Geometry: final body of the model. Coordinates: model frame, mm. A direction names the side the tool comes from. Round coordinates to 2 decimals unless told otherwise and drop trailing zeros. Loops run counter-clockwise (first coordinate to the right, second up) from the corner with the lowest first, then second, coordinate; pieces in that order, holes last. Notation, with made-up numbers: M 75.25,-38.5 L 107.25,-38.5 A33 ccw 107.25,-4.5 Z; hole C 79,75.25 d6. An arc over 180 degrees is marked long. Answer as a JSON object with one key per item and string values.
```python
from build123d import *

# Parameters (mm, degrees)
F1_DEPTH = 100
F2_W     = 980
F2_H     = 769.125695
F3_DEPTH = 250
F4_W     = 244.644434
F4_H     = 193.814576
F4_W_2   = 221.683964
F4_H_2   = 205.729261
F5_DEPTH = 600


with BuildPart() as f1:
    # F0 (on Top) → F1 (new body)
    with BuildSketch(Plane.XY):
        Polygon((-780, 0), (0, 0), (-18.731487, 589.702579), (-748.441424, 569.125695), align=None)
    extrude(amount=F1_DEPTH)

    # F2 (on face) → F3 (join)
    with BuildSketch(Plane(origin=(0, 0, 0), x_dir=(1, 0, 0), z_dir=(0, 0, -1))):
        with Locations((-390, -284.562847)):
            Rectangle(F2_W, F2_H)
    extrude(amount=F3_DEPTH)

    # F4 (on face) → F5 (cut)
    with BuildSketch(Plane.XY.offset(100)):
        with Locations((-537.912771, 294.744283)):
            Rectangle(F4_W, F4_H)
        with Locations((-218.167432, 298.055314)):
            Rectangle(F4_W_2, F4_H_2)
    extrude(amount=-F5_DEPTH, mode=Mode.SUBTRACT)


solid = f1.part
```
1) First-contact query: pin 1 (6 mm diameter, centred on y = 254.5, z = 60.5, fed in from +X); pin 2 (10 mm diameter, centred on y = 201, z = 47.5, fed in from -X); pin 3 (4 mm diameter, centred on y = -1.5, z = 21, fed in from -X). Flat tips, straight axial feed; report the tip coordinate or a pass-through.
Geometry results:
{"pin 1": "x = -7.99", "pin 2": "x = -769.13", "pin 3": "x = -780"}
2) Cut plane C-C on y = 295. Return the cut outline in (x, z), and give its area (3 significant figures).
Geometry results:
{"outline": "M -880,-250 L -660.23,-250 L -660.23,100 L -763.64,100 L -763.64,0 L -880,0 Z; M -415.59,-250 L -329.01,-250 L -329.01,100 L -415.59,100 Z; M -107.33,-250 L 100,-250 L 100,0 L -9.37,0 L -9.37,100 L -107.33,100 Z", "area": "157,000 mm2"}
3) Set-up query: faces 5 (the face through (-395, 0, 49)), 6 (the face through (-764, 288.55, 49.3)), 7 (the face through (-660.235, 293, -73)), 8 (the face through (100, 290, -123)), 9 (the face through (-397, -100, -123)). Return all of +Z, -Z, +X, -X, +Y, -Y with unobstructed straight access to the full face (end or side cutting, diameter ignored); none if empty.
Geometry results:
{"face 5": "+Z, +X, -X, -Y", "face 6": "+Z, -X, +Y", "face 7": "+Z, -Z", "face 8": "+Z, -Z, +X, +Y, -Y", "face 9": "+Z, -Z, +X, -X, -Y"}
4) Cut plane D-D on x = -728. Return the cut outline in (y, z), and give its area (3 significant figures).
Geometry results:
{"outline": "M -100,-250 L 669.13,-250 L 669.13,0 L 569.7,0 L 569.7,100 L 0,100 L 0,0 L -100,0 Z", "area": "249,000 mm2"}
5) Cut plane A-A on z = -227. Return the cut outline in (x, y), and give its area (3 significant figures).
Geometry results:
{"outline": "M -880,-100 L 100,-100 L 100,669.13 L -880,669.13 Z; hole M -660.23,197.84 L -415.59,197.84 L -415.59,391.65 L -660.23,391.65 Z; hole M -329.01,195.19 L -107.33,195.19 L -107.33,400.92 L -329.01,400.92 Z", "area": "661,000 mm2"}
6) Pull-direction query (Y, two-part tool) for faces 1 (the face through (-397, 669.126, -123)), 2 (the face through (-540, 391.652, -73)), 3 (the face through (-880, 290, -123)), 4 (the face through (-107.325, 297, -73)); classes: +Y half, -Y half, draft (parallel to the pull), parting line (faces both ways), or undercut.
Geometry results:
{"face 1": "+Y half", "face 2": "undercut", "face 3": "draft", "face 4": "undercut"}
7) Line query: probe 1 along X at (y, z) = (382, -151.5); probe 2 along Y at (x, z) = (-596, -81); probe 3 along Y at (x, z) = (-248, -53.5). Output: solid intervals per line, ascending.
Geometry results:
{"probe 1": "-880 to -660.23, -415.59 to -329.01, -107.33 to 100", "probe 2": "-100 to 197.84, 391.65 to 669.13", "probe 3": "-100 to 195.19, 400.92 to 669.13"}
8) Cut plane B-B on x = -627. Return the cut outline in (y, z).
Geometry results:
{"outline": "M -100,-250 L 197.84,-250 L 197.84,100 L 0,100 L 0,0 L -100,0 Z; M 391.65,-250 L 669.13,-250 L 669.13,0 L 572.55,0 L 572.55,100 L 391.65,100 Z"}
